Geometry: final body of the model. Coordinates: model frame, mm. Face numbers are marked on the shaded views. A direction names the side the tool comes from. Give positions to 0.01 mm unless a question says otherwise; leave off trailing zeros. Loops run counter-clockwise (first coordinate to the right, second up) from the corner with the lowest first, then second, coordinate; pieces in that order, holes last. Notation, with made-up numbers: (43.5, 20.5) - (75.5, 20.5) arc R28 cw to (75.5, 39.5) - close; hole circle Ø9 at (51.25, -5). An arc over 180 degrees is marked (long way). Use one line per item in the form item = value.
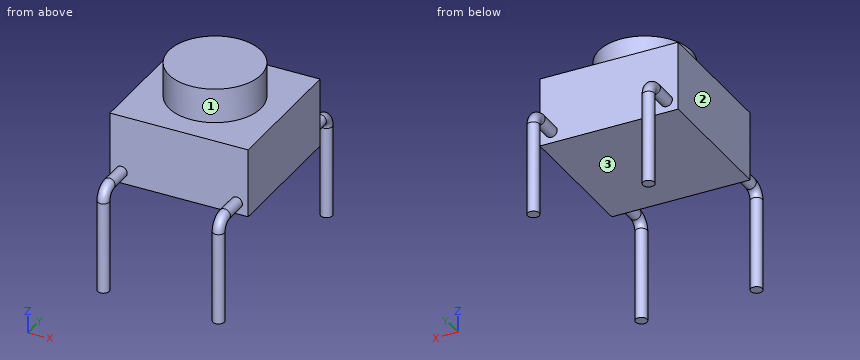
```python
from build123d import *

# Parameters (mm, degrees)
F0_W     = 6
F0_H     = 6
F1_DEPTH = 3
F2_R     = 2
F3_DEPTH = 1.5
F4_R     = 0.25


# Not quite as in the source:
# - a pattern or mirror of a feature is missing from the dataset's text; its kind, count and spacing are read off the source's solid


with BuildPart() as f1:
    # F0 (on Top) → F1 (new body)
    with BuildSketch(Plane.XY):
        Rectangle(F0_W, F0_H)
    extrude(amount=F1_DEPTH)

    # F2 (on face) → F3 (join)
    with BuildSketch(Plane.XY.offset(3)):
        Circle(F2_R)
    extrude(amount=F3_DEPTH)

    # F6: sweep along a path in F5
    with BuildLine(Plane(origin=(-3, 0, 0), x_dir=(0, -1, 0), z_dir=(-1, 0, 0))) as f6_path:
        Line((3, 0.7), (4, 0.7))
        ThreePointArc((4, 0.7), (4.4949747468, 0.4949747468), (4.7, 0))
        Line((4.7, 0), (4.7, -4))
    # F4 (on face) → F6 (sweep)
    with BuildSketch(Plane.XZ.offset(3)):
        with Locations((-2.5, 0.5)):
            Circle(F4_R)
        with Locations((2.5, 0.5)):
            Circle(F4_R)
    f6 = sweep(path=f6_path.line)

    # F6_copies: F6 across plane
    add(f6.mirror(Plane.ZX))


solid = f1.part
```
(1) Access query for the marked faces 1, 2 and 3. Directions: +Z, -Z, +X, -X, +Y, -Y. A direction counts if a zero-diameter tool reaches every point of the face in a straight line with its end or side. Return the directions, or none.
Solution:
face_1 = +Z
face_2 = +Z, -Z, -X, +Y, -Y
face_3 = -Z, +X, -X
(2) Cut plane D-D (z = 2). Return the cut outline in (x, y).
Solution:
outline = (-3, -3) - (3, -3) - (3, 3) - (-3, 3) - close
(3) Pin query (flat end, axial travel): P1, Ø1.5, axis at x = -1, z = 1, coming from the -Y side; P2, Ø3, axis at x = 0.5, y = 1.5, coming from the -Z side; P3, Ø1.5, axis at x = 1.5, z = 1, coming from the +Y side. Return the tip coordinate at first contact, or that it passes through.
Solution:
P1 = -3
P2 = 0
P3 = 3
(4) Material intervals for L1, parallel to Y at x = 2.5, z = -1; L2, parallel to Z at x = 1.75, y = 2.5; L3, parallel to Z at x = -0.9, y = 1.25, sorted ascending. Write a range as from..to.
Solution:
L1 = -4.75..-4.25, 4.25..4.75
L2 = 0..3
L3 = 0..4.5
(5) Cut plane C-C (y = 0). Return the cut outline in (x, z).
Solution:
outline = (-3, 0) - (3, 0) - (3, 3) - (2, 3) - (2, 4.5) - (-2, 4.5) - (-2, 3) - (-3, 3) - close
(6) Cut plane B-B (z = -2.5). Return the cut outline in (x, y), plus the area to 3 significant figures.
Solution:
outline = circle Ø0.5 at (-2.5, -4.5); circle Ø0.5 at (-2.5, 4.5); circle Ø0.5 at (2.5, -4.5); circle Ø0.5 at (2.5, 4.5)
area = 0.785 mm2
(7) Cut plane A-A (x = 2.5). Return the cut outline in (y, z), plus the area to 3 significant figures.
Solution:
outline = (-4.75, -4) - (-4.25, -4) - (-4.25, 0) arc R0.25 cw to (-4, 0.25) - (-3, 0.25) - (-3, 0) - (3, 0) - (3, 0.25) - (4, 0.25) arc R0.25 cw to (4.25, 0) - (4.25, -4) - (4.75, -4) - (4.75, 0) arc R0.75 ccw to (4, 0.75) - (3, 0.75) - (3, 3) - (-3, 3) - (-3, 0.75) - (-4, 0.75) arc R0.75 ccw to (-4.75, 0) - close
area = 23.8 mm2
